Autodesk Inventor part; units mm, degrees
ref_plane "YZ Plane" through (0, 0, 0) normal (1, 0, 0) x (0, 1, 0)
ref_plane "XZ Plane" through (0, 0, 0) normal (0, 1, 0) x (-1, 0, 0)
ref_plane "XY Plane" through (0, 0, 0) normal (0, 0, 1) x (1, 0, 0)
sketch "Sketch1" plane through (0, 0, 0) normal (0, 0, 1) x (1, 0, 0)
  line L0 (-12.273, 14.9908) -> (-12.273, -33.0092)
  line L1 (-12.273, -33.0092) -> (22.727, -33.0092)
  line L2 (53.727, -23.0092) -> (53.727, 4.9908)
  line L3 (-12.273, 14.9908) -> (22.727, 14.9908)
  line L4 (22.727, 14.9908) -> (22.727, 4.9908)
  line L5 (22.727, 4.9908) -> (53.727, 4.9908)
  line L6 (22.727, 4.9908) -> (22.727, -33.0092)
  line L7 (53.727, -23.0092) -> (22.727, -23.0092)
  line L8 (22.727, -33.0092) -> (53.727, -23.0092)
  line L9 (53.727, 4.9908) -> (22.727, 14.9908)
  line L10 (29.727, 0.9908) -> (27.727, 0.9908) construction
  line L11 (29.727, 2.4908) -> (27.727, 2.4908)
  line L12 (27.727, -0.5092) -> (29.727, -0.5092)
  arc A0 (29.727, -0.5092) -> (29.727, 2.4908) centre (29.727, 0.9908) ccw
  arc A1 (27.727, 2.4908) -> (27.727, -0.5092) centre (27.727, 0.9908) ccw
  line L13 (49.727, 0.9908) -> (47.727, 0.9908) construction
  line L14 (49.727, 2.4908) -> (47.727, 2.4908)
  line L15 (47.727, -0.5092) -> (49.727, -0.5092)
  arc A2 (49.727, -0.5092) -> (49.727, 2.4908) centre (49.727, 0.9908) ccw
  arc A3 (47.727, 2.4908) -> (47.727, -0.5092) centre (47.727, 0.9908) ccw
  line L16 (29.727, -19.0092) -> (27.727, -19.0092) construction
  line L17 (29.727, -17.5092) -> (27.727, -17.5092)
  line L18 (27.727, -20.5092) -> (29.727, -20.5092)
  arc A4 (29.727, -20.5092) -> (29.727, -17.5092) centre (29.727, -19.0092) ccw
  arc A5 (27.727, -17.5092) -> (27.727, -20.5092) centre (27.727, -19.0092) ccw
  line L19 (49.727, -19.0092) -> (47.727, -19.0092) construction
  line L20 (49.727, -17.5092) -> (47.727, -17.5092)
  line L21 (47.727, -20.5092) -> (49.727, -20.5092)
  arc A6 (49.727, -20.5092) -> (49.727, -17.5092) centre (49.727, -19.0092) ccw
  arc A7 (47.727, -17.5092) -> (47.727, -20.5092) centre (47.727, -19.0092) ccw
  line L22 (39.727, -9.0092) -> (37.727, -9.0092) construction
  line L23 (39.727, -2.5092) -> (37.727, -2.5092)
  line L24 (37.727, -15.5092) -> (39.727, -15.5092)
  arc A8 (39.727, -15.5092) -> (39.727, -2.5092) centre (39.727, -9.0092) ccw
  arc A9 (37.727, -2.5092) -> (37.727, -15.5092) centre (37.727, -9.0092) ccw
  point P0 (0, 0)
  point P1 (-7.273, 10.4908)
  point P2 (-7.273, -9.0092)
  point P3 (-7.273, -28.5092)
  point P4 (17.727, 10.4908)
  point P5 (17.727, -9.0092)
  point P6 (17.727, -28.5092)
  point P7 (28.727, 0.9908)
  point P8 (48.727, 0.9908)
  point P9 (28.727, -19.0092)
  point P10 (48.727, -19.0092)
  point P11 (38.727, -9.0092)
  dimension "d0" = 48
  dimension "d2" = 28
  dimension "d3" = 35
  dimension "d4" = 5
  dimension "d5" = 5
  dimension "d6" = 4.5
  dimension "d7" = 4.5
  dimension "d8" = 24
  dimension "d9" = 20
  dimension "d10" = 20
  dimension "d13" = 10
  dimension "d14" = 10
  dimension "d44" = 4
  dimension "d45" = 66
  dimension "d46" = 4
  dimension "d47" = 10
  dimension "d53" = 31
  dimension "d54" = 2
  dimension "d55" = 3
  dimension "d56" = 2
  dimension "d57" = 3
  dimension "d58" = 2
  dimension "d59" = 3
  dimension "d60" = 2
  dimension "d61" = 3
  dimension "d62" = 2
  dimension "d63" = 13
extrude "Extrusion1" add sketch "Sketch1" along normal blind 2.5
hole "Hole1" at (-7.273, 10.4908, 0) at (-7.273, -9.0092, 0) at (-7.273, -28.5092, 0) at (17.727, 10.4908, 0) at (17.727, -9.0092, 0) at (17.727, -28.5092, 0) direction (0, 0, 1) diameter 3 end through all
chamfer "Chamfer3" distance 3 angle 45 2 edges at (-12.273, -33.0092, 1.25) (-12.273, 14.9908, 1.25)
equation "\"d10\" = d9"
equation "\"d13\" = 0.5 * d9"
equation "\"d14\" = d13"
equation "\"d44\" = d46"
equation "\"d46\" = -0.5 * d9 + 0.5 * d2"
equation "\"d47\" = -0.5 * d2 + 0.5 * d0"
properties part number "LC_ALU_3mm_X_axis_belt_idler_mount_plate" material "Aluminum 6061-AHC"
Can you work these out from the model? Positions are in its coordinate system, mm. Give positions to 0.01 mm unless a question says otherwise; leave off trailing zeros. Order: outer loops, then holes, each group sorted by start corner. A loop starts at its lowest first (then second) coordinate and runs counter-clockwise, first axis right, second up. Notation, with made-up numbers: (-4.75, 29) - (12.25, 29) arc R20 cw to (12.25, 57) - close; hole circle Ø8 at (61, 89). An arc over 180 degrees is marked (long way). Use a Markdown table: item, result. Add a question column.
Q1. Please list where these lines run through material, in increasing order: line 1 along X through (y, z) = (1, 0.35); line 2 along X through (y, z) = (-9, 0.7); line 3 along Y through (x, z) = (27.5, 1.4).
Q2. If we mould it in two halves opening along X, with no side actions, what happens to faces 1 (the flat face through (38.01, -28.08, 1.23)), 2 (the flat face through (7, -33.009, 1)), 3 (the flat face through (29, -17.509, 1))? For each: released by +X, released by -X, zero draft, split by the parting line, or undercut.
Q3. If we section it at B-B on z = 1.6: Count the separate pieces of the cut face and the enclosed holes in it, plus the area to 3 significant figures.
Q4. If we section it at A-A on y = -5.5: Write out the boundary of the cut face in (x, z), plus the area to 3 significant figures.
Q5. If we section it at D-D on y = -24.5: Write out the boundary of the cut face in (x, z), plus the area to 3 significant figures.
Q6. I'm going to push flat-ended pins straight in: pin 1 (0.6 mm diameter, centred on x = 48.5, z = 1, fed in from +Y); pin 2 (1 mm diameter, centred on x = 29, z = 1.5, fed in from +Y); pin 3 (0.6 mm diameter, centred on x = 28.5, z = 1, fed in from -Y); pin 4 (1.8 mm diameter, centred on x = -7.27, y = 10.49, fed in from +Z). Where does each tip first touch, or does it pass through?
Q7. If we section it at C-C on y = -14: Write out the boundary of the cut face in (x, z), plus the area to 3 significant figures.
Answers follow:
| question | item | result |
|---|---|---|
| 1 | line 1 | x = -12.27 to 26.23, 31.23 to 46.23, 51.23 to 53.73 |
| 1 | line 2 | x = -12.27 to -8.77, -5.77 to 16.23, 19.23 to 31.23, 46.23 to 53.73 |
| 1 | line 3 | y = -31.47 to -20.49, -17.53 to -0.49, 2.47 to 13.45 |
| 2 | face 1 | released by +X |
| 2 | face 2 | zero draft |
| 2 | face 3 | undercut |
| 3 | separate pieces | 1 |
| 3 | enclosed holes | 11 |
| 3 | area | 2,600 mm^2 |
| 4 | outline | (-12.27, 0) - (32.26, 0) - (32.26, 2.5) - (-12.27, 2.5) - close; (45.2, 0) - (53.73, 0) - (53.73, 2.5) - (45.2, 2.5) - close |
| 4 | area | 133 mm^2 |
| 5 | outline | (-12.27, 0) - (49.11, 0) - (49.11, 2.5) - (-12.27, 2.5) - close |
| 5 | area | 153 mm^2 |
| 6 | pin 1 | stops at y = 6.77 |
| 6 | pin 2 | stops at y = 13.13 |
| 6 | pin 3 | stops at y = -31.24 |
| 6 | pin 4 | passes through |
| 7 | outline | (-12.27, 0) - (33.56, 0) - (33.56, 2.5) - (-12.27, 2.5) - close; (43.89, 0) - (53.73, 0) - (53.73, 2.5) - (43.89, 2.5) - close |
| 7 | area | 139 mm^2 |
